Autodesk Inventor part; units mm, degrees
ref_plane "YZ Plane" through (0, 0, 0) normal (1, 0, 0) x (0, 1, 0)
ref_plane "XZ Plane" through (0, 0, 0) normal (0, 1, 0) x (-1, 0, 0)
ref_plane "XY Plane" through (0, 0, 0) normal (0, 0, 1) x (1, 0, 0)
sketch "Sketch1" plane through (0, 0, 0) normal (0, 0, 1) x (1, 0, 0)
  line L0 (-27.45, -52.45) -> (27.45, -52.45) construction
  line L1 (52.45, -27.45) -> (52.45, 27.45) construction
  line L2 (27.45, 52.45) -> (-27.45, 52.45) construction
  line L3 (-52.45, 27.45) -> (-52.45, -27.45) construction
  line L4 (-52.45, -52.45) -> (52.45, 52.45) construction
  line L5 (52.45, -52.45) -> (-52.45, 52.45) construction
  arc A0 (-27.45, 52.45) -> (-52.45, 27.45) centre (-27.45, 27.45) ccw construction
  arc A1 (-52.45, -27.45) -> (-27.45, -52.45) centre (-27.45, -27.45) ccw construction
  arc A2 (27.45, -52.45) -> (52.45, -27.45) centre (27.45, -27.45) ccw construction
  arc A3 (52.45, 27.45) -> (27.45, 52.45) centre (27.45, 27.45) ccw construction
  line L6 (47.45, 27.45) -> (47.45, -27.45)
  arc A4 (27.45, -47.45) -> (47.45, -27.45) centre (27.45, -27.45) ccw
  line L7 (27.45, -47.45) -> (-27.45, -47.45)
  arc A5 (-47.45, -27.45) -> (-27.45, -47.45) centre (-27.45, -27.45) ccw
  line L8 (-47.45, -27.45) -> (-47.45, 27.45)
  arc A6 (-27.45, 47.45) -> (-47.45, 27.45) centre (-27.45, 27.45) ccw
  line L9 (-27.45, 47.45) -> (27.45, 47.45)
  arc A7 (47.45, 27.45) -> (27.45, 47.45) centre (27.45, 27.45) ccw
  line L10 (-35, 35) -> (35, 35) construction
  line L11 (35, 35) -> (35, -35) construction
  line L12 (35, -35) -> (-35, -35) construction
  line L13 (-35, -35) -> (-35, 35) construction
  line L14 (-35, 35) -> (35, -35) construction
  line L15 (35, 35) -> (-35, -35) construction
  circle A8 centre (35, 35) radius 4
  circle A9 centre (35, -35) radius 4
  circle A10 centre (-35, -35) radius 4
  circle A11 centre (-35, 35) radius 4
  point P0 (0, 0)
  dimension "d0" = 104.9
  dimension "d1" = 104.9
  dimension "d2" = 25
  dimension "d6" = 5
  dimension "d12" = 70
  dimension "d13" = 8
extrude "Extrusion1" add sketch "Sketch1" along normal blind 6
sketch "Sketch2" plane through (0, 0, 6) normal (0, 0, 1) x (1, 0, 0)
  line L0 (-30, 30) -> (30, 30)
  line L1 (30, 30) -> (30, -30)
  line L2 (30, -30) -> (-30, -30)
  line L3 (-30, 30) -> (30, -30) construction
  line L4 (30, 30) -> (-30, -30) construction
  line L5 (-64.9, 2) -> (-30, 2)
  line L6 (-30, -2) -> (-64.9, -2)
  line L7 (-64.9, -2) -> (-64.9, 2)
  line L8 (-47.45, 27.45) -> (-47.45, -27.45)
  line L9 (-64.9, 2) -> (-30, -2) construction
  line L10 (-30, 2) -> (-64.9, -2) construction
  line L11 (-30, -30) -> (-30, -2)
  line L12 (-30, 2) -> (-30, 30)
  point P0 (0, 0)
  point P1 (-47.45, 0)
  dimension "d7" = 4
  dimension "d8" = 60
  dimension "d9" = 60
extrude "Extrusion2" cut sketch "Sketch2" against normal blind 10
fillet "Fillet1" radius 5 4 edges at (30, 30, 3) (-30, 30, 3) (30, -30, 3) (-30, -30, 3)
equation "\"d1\" = d0"
equation "\"d8\" = d9"
properties part number "NewFront_E"
Part model, mm, in its own coordinate system. A direction names the side the tool comes from. Give positions to 0.01 mm unless a question says otherwise; leave off trailing zeros. Loops run counter-clockwise (first coordinate to the right, second up) from the corner with the lowest first, then second, coordinate; pieces in that order, holes last. Notation, with made-up numbers: (46.25, 38) -> (65.25, 38) arc R25 ccw to (65.25, 66) -> close; hole circle Ø9 at (7, 23). An arc over 180 degrees is marked (long way). Write each question's results on one line, items separated by ' | '. Start each with the question number.
Q1. Band-saw the part on B-B on z = 4.5. List the corners of the cut face in (x, y), plus the area to 3 significant figures.
Q2. Pin check, flat tips, straight feed: P1, Ø6.5, axis at x = -35, y = -35, coming from the +Z side; P2, Ø3, axis at x = -42.5, z = 3.5, coming from the +Y side. Stop position of each tip, or through.
Q3. Which spindle directions (+Z, -Z, +X, -X, +Y, -Y) get a long thin tool onto all of the face, cutting with end or side? Do faces 1 (the face through (0, 47.45, 3)), 2 (the face through (28, 29, 3)). Say none if no direction does.
Q4. Band-saw the part on C-C on y = -35. List the corners of the cut face in (x, z), plus the area to 3 significant figures.
Q5. Wall check: L1, parallel to Y at x = 23.5, z = 3.25; L2, parallel to Y at x = -37, z = 2.4; L3, parallel to Y at x = 35, z = 3.3. Give the ranges that are in metal, low to high.
Q6. Pull direction X, two halves, no side cores. Call faces 3 (the face through (-41.747, 41.436, 2.958)), 4 (the face through (30, 0, 3)), 5 (the face through (-39, -2, 3)), 6 (the face through (41.747, -41.436, 2.958)): +X half, -X half, draft (parallel to the pull), parting line (faces both ways), or undercut.
Q7. Band-saw the part on A-A on x = 12. List the corners of the cut face in (y, z), plus the area to 3 significant figures.
Results are:
1) outline: (-47.45, -27.45) arc R20 ccw to (-27.45, -47.45) -> (27.45, -47.45) arc R20 ccw to (47.45, -27.45) -> (47.45, 27.45) arc R20 ccw to (27.45, 47.45) -> (-27.45, 47.45) arc R20 ccw to (-47.45, 27.45) -> (-47.45, 2) -> (-30, 2) -> (-30, 25) arc R5 cw to (-25, 30) -> (25, 30) arc R5 cw to (30, 25) -> (30, -25) arc R5 cw to (25, -30) -> (-25, -30) arc R5 cw to (-30, -25) -> (-30, -2) -> (-47.45, -2) -> close; hole circle Ø8 at (-35, -35); hole circle Ø8 at (-35, 35); hole circle Ø8 at (35, -35); hole circle Ø8 at (35, 35) | area: 4,810 mm²
2) P1: passes through | P2: stops at y = 42.16
3) face 1: +Z, -Z, +X, -X, +Y | face 2: +Z, -Z
4) outline: (-45.97, 0) -> (-39, 0) -> (-39, 6) -> (-45.97, 6) -> close; (-31, 0) -> (31, 0) -> (31, 6) -> (-31, 6) -> close; (39, 0) -> (45.97, 0) -> (45.97, 6) -> (39, 6) -> close | area: 456 mm²
5) L1: y = -47.45 to -30, 30 to 47.45 | L2: y = -45.02 to -38.46, -31.54 to -2, 2 to 31.54, 38.46 to 45.02 | L3: y = -45.97 to -39, -31 to 31, 39 to 45.97
6) face 3: -X half | face 4: undercut | face 5: draft | face 6: +X half
7) outline: (-47.45, 0) -> (-30, 0) -> (-30, 6) -> (-47.45, 6) -> close; (30, 0) -> (47.45, 0) -> (47.45, 6) -> (30, 6) -> close | area: 209 mm²
